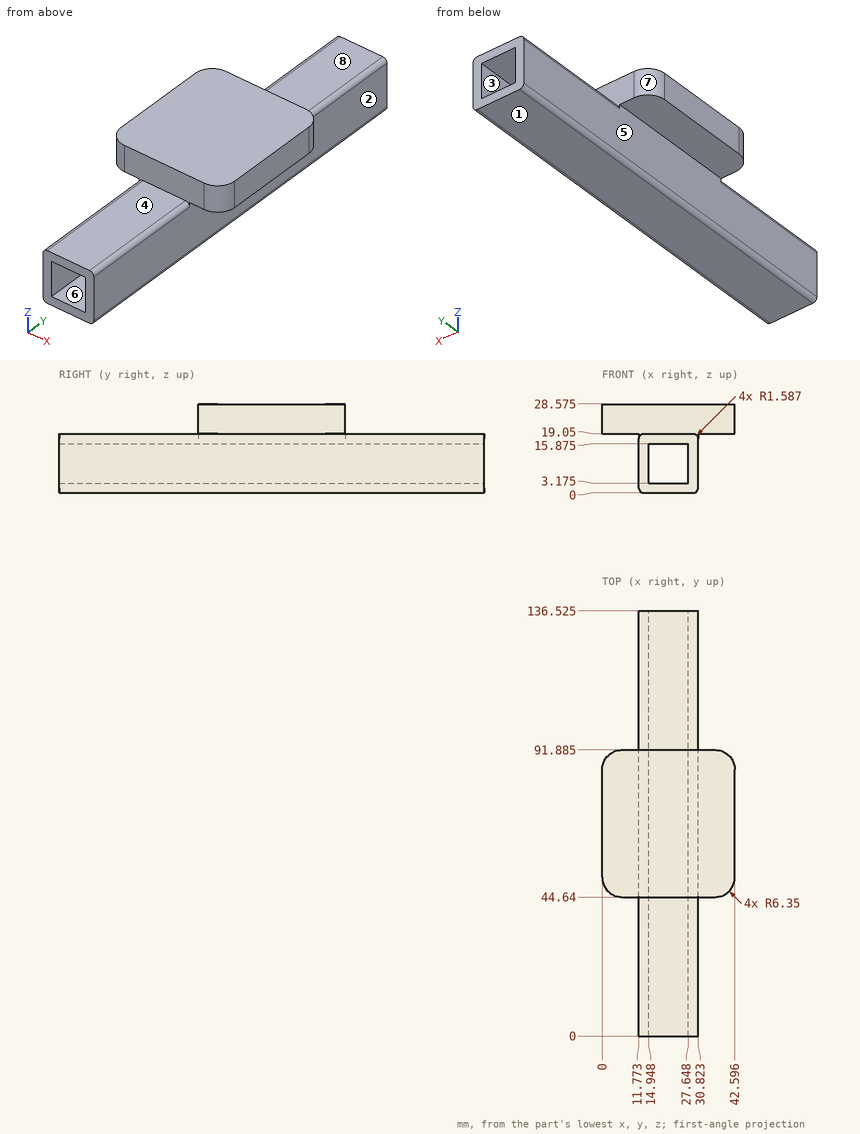
Can you work these out from the drawing? Everything is in mm from the part's minimum corner. A direction names the side the tool comes from. Round coordinates to 2 decimals unless told otherwise and drop trailing zeros. Write each question's results on one line, items separated by ' | '. Start each with the question number.
1) Which directions (+Z, -Z, +X, -X, +Y, -Y) give clear straight access to the entire face, cutting with the end or side of a thin tool? Please do the marked faces 4, 5, 6, 7 and 8.
2) Please list where these lines run through material, in increasing order: line 1 (Z direction, x = 17, y = 85.5) (1 decimal); line 2 (X direction, y = 18, z = 10.25); line 3 (Y direction, x = 12.5, z = 25.25) (1 decimal).
3) For pin 1 Ø13 at (x, y) = (6, 66.5) entering from -Z; pin 2 Ø9.5 at (x, y) = (37, 75.5) entering from -Z; pin 3 Ø14 at (y, z) = (34.5, 11.5) entering from -X; pin 4 Ø3 at (x, y) = (8, 94.5) entering from -Z, each with a flat end and sliding along its axis, tell me the tip position at first contact or that it passes through.
4) We'd pull the mould along X, two halves only. Please class the marked faces 1, 2 and 3: released by +X, released by -X, zero draft, split by the parting line, or undercut.
Here are the results:
1) face 4: +Z, +X, -X, -Y | face 5: -Z, -X, +Y, -Y | face 6: +Y, -Y | face 7: +Z, -Z, -X, +Y | face 8: +Z, +X, -X, +Y
2) line 1: z = 0 to 3.2, 15.9 to 28.6 | line 2: x = 11.77 to 14.95, 27.65 to 30.82 | line 3: y = 44.6 to 91.9
3) pin 1: stops at z = 0.25 | pin 2: stops at z = 19.05 | pin 3: stops at x = 11.77 | pin 4: passes through
4) face 1: zero draft | face 2: released by +X | face 3: undercut
